Design review of the part built by this model. Coordinates are the model's own, in mm. A direction names the side the tool comes from. Give positions to 0.01 mm unless a question says otherwise; leave off trailing zeros. Loops run counter-clockwise (first coordinate to the right, second up) from the corner with the lowest first, then second, coordinate; pieces in that order, holes last. Notation, with made-up numbers: (45.25, 36) - (78.25, 36) arc R21 cw to (78.25, 57) - close; hole circle Ø4 at (24.5, 75). An arc over 180 degrees is marked (long way). Write each question's results on one line, items separated by ' | '.
```python
from build123d import *

# Parameters (mm, degrees)
BOSS_EXTRUDE1_DEPTH      = 20
BOSS_EXTRUDE2_DEPTH      = 65
BOSS_EXTRUDE2_DEPTH_BACK = 20
SKETCH3_R                = 31
SKETCH3_R_2              = 12.5
SKETCH6_R                = 20
CUT_EXTRUDE1_DEPTH       = 26
SKETCH8_R                = 12.5
CUT_EXTRUDE2_DEPTH       = 20
SKETCH9_R                = 3
CUT_EXTRUDE3_DEPTH       = 33


with BuildPart() as part:
    # Sketch2 → Boss-Extrude1 (new body)
    with BuildSketch(Plane.XY):
        with BuildLine():
            Line((0, 0), (56.291651246, -32.5))
            ThreePointArc((56.291651246, -32.5), (64.9518339, -2.501853916), (58.624860802, 28.073576473))
            Line((58.624860802, 28.073576473), (45.634479745, 20.573576473))
            Line((45.634479745, 20.573576473), (40.634479745, 29.233830511))
            Line((40.634479745, 29.233830511), (53.624860802, 36.733830511))
            ThreePointArc((53.624860802, 36.733830511), (32.5, 56.291651246), (5, 64.807406984))
            Line((5, 64.807406984), (5, 49.807406984))
            Line((5, 49.807406984), (-5, 49.807406984))
            Line((-5, 49.807406984), (-5, 64.807406984))
            ThreePointArc((-5, 64.807406984), (-32.5, 56.291651246), (-53.624860802, 36.733830511))
            Line((-53.624860802, 36.733830511), (-40.634479745, 29.233830511))
            Line((-40.634479745, 29.233830511), (-45.634479745, 20.573576473))
            Line((-45.634479745, 20.573576473), (-58.624860802, 28.073576473))
            ThreePointArc((-58.624860802, 28.073576473), (-64.9518339, -2.501853916), (-56.291651246, -32.5))
            Line((-56.291651246, -32.5), (0, 0))
        make_face()
    extrude(amount=BOSS_EXTRUDE1_DEPTH)

    # Sketch3 → Boss-Extrude2 (add, two sides: drawn at the far end of the back side and taken through both)
    with BuildSketch(Plane.XY.offset(20).offset(-BOSS_EXTRUDE2_DEPTH_BACK)):
        Circle(SKETCH3_R)
        Circle(SKETCH3_R_2, mode=Mode.SUBTRACT)
    extrude(amount=BOSS_EXTRUDE2_DEPTH + BOSS_EXTRUDE2_DEPTH_BACK)

    # Cut-Sweep1: sweep along a curve in space
    with BuildLine() as cut_sweep1_path:
        ThreePointArc((31, 0, 85), (21.920310217, 21.920310217, 85), (0, 31, 85))
        ThreePointArc((0, 31, 85), (-21.920310217, 21.920310217, 85), (-31, 0, 85))
        ThreePointArc((-31, 0, 85), (-21.920310217, -21.920310217, 85), (0, -31, 85))
        ThreePointArc((0, -31, 85), (21.920310217, -21.920310217, 85), (31, 0, 85))
    # Sketch5 → Cut-Sweep1 (sweep, cut)
    with BuildSketch(Plane(origin=(0, 0, 0), x_dir=(0, 0, -1), z_dir=(1, 0, 0))):
        Polygon((-85, 31), (-73, 31), (-85, 24.07179677), align=None)
    sweep(path=cut_sweep1_path.line, mode=Mode.SUBTRACT)

    # Sketch6 → Cut-Extrude1 (cut)
    with BuildSketch(Plane.XY.offset(85)):
        Circle(SKETCH6_R)
    extrude(amount=-CUT_EXTRUDE1_DEPTH, mode=Mode.SUBTRACT)

    # Sketch8 → Cut-Extrude2 (cut)
    with BuildSketch(Plane.XY.offset(20)):
        Circle(SKETCH8_R)
    extrude(amount=-CUT_EXTRUDE2_DEPTH, mode=Mode.SUBTRACT)

    # Sketch9 → Cut-Extrude3 (cut)
    with BuildSketch(Plane(origin=(0, 0, 0), x_dir=(1, 0, 0), z_dir=(0, 1, 0))):
        with Locations(Location((0, -33, 0), (0, 0, 90))):
            Circle(SKETCH9_R)
    extrude(amount=CUT_EXTRUDE3_DEPTH, mode=Mode.SUBTRACT)


solid = part.part
```
Item 1: Draft analysis for pull direction X (two halves, no side actions). For faces 1 (the face through (-15, 28, 20)), 2 (the face through (-32.15, 56.49, 9.86)), 3 (the face through (-43.1, 24.96, 9.86)), state which applies: +X half, -X half, draft (parallel to the pull), parting line (faces both ways), or undercut.
Output values:
face 1: draft | face 2: -X half | face 3: undercut
Item 2: Wall thickness on probe 1 along X at (y, z) = (-18.5, 17); probe 2 along Y at (x, z) = (0, 14); probe 3 along Z at (x, y) = (45, 1): over which ranges is each line inside the solid? List them lowest first.
Output values:
probe 1: x = -62.31 to -32.04, -24.87 to 24.87, 32.04 to 62.31 | probe 2: y = -31 to -12.5, 12.5 to 49.81 | probe 3: z = 0 to 20
Item 3: Tool access review of faces 4 (the face through (-4.336, -19.524, 72.182)), 5 (the face through (41.4, -23.9, 9.9)), 6 (the face through (52.221, 24.376, 9.86)): name each direction out of +Z, -Z, +X, -X, +Y, -Y from which nothing blocks a thin tool from reaching the whole face with its end or side.
Output values:
face 4: +Z | face 5: +Z, -Z, -Y | face 6: +Z, -Z
Item 4: We need section A-A on z = 7. Give the boundary of the cut face in (x, y).
Output values:
outline: (-58.62, 28.07) arc R65 ccw to (-56.29, -32.5) - (-26.85, -15.5) arc R31 ccw to (26.85, -15.5) - (56.29, -32.5) arc R65 ccw to (58.62, 28.07) - (45.63, 20.57) - (40.63, 29.23) - (53.62, 36.73) arc R65 ccw to (5, 64.81) - (5, 49.81) - (-5, 49.81) - (-5, 64.81) arc R65 ccw to (-53.62, 36.73) - (-40.63, 29.23) - (-45.63, 20.57) - close; hole circle Ø25 at (0, 0)
Item 5: Clearance check with flat-ended pins moving along their axes: P1, Ø8, axis at x = -35.5, y = 10.5, coming from the +Z side; P2, Ø8, axis at x = -2.5, z = 12.5, coming from the +Y side; P3, Ø16.5, axis at y = 59, z = 12, coming from the -X side. State where each tip first meets the part, or that it passes through.
Output values:
P1: stops at z = 20 | P2: stops at y = 64.81 | P3: stops at x = -40.61
Item 6: We need section B-B on x = -51. Give the boundary of the cut face in (y, z), then the cut area to 3 significant figures.
Output values:
outline: (-29.44, 0) - (23.67, 0) - (23.67, 20) - (-29.44, 20) - close; (35.22, 0) - (40.3, 0) - (40.3, 20) - (35.22, 20) - close | area: 1,160 mm²
Item 7: We need section D-D on x = 38. Give the boundary of the cut face in (y, z), then the cut area to 3 significant figures.
Output values:
outline: (-21.94, 0) - (52.74, 0) - (52.74, 20) - (-21.94, 20) - close | area: 1,490 mm²
Item 8: We need section C-C on y = 53. Give the boundary of the cut face in (x, z), then the cut area to 3 significant figures.
Output values:
outline: (-37.63, 0) - (-5, 0) - (-5, 20) - (-37.63, 20) - close; (5, 0) - (37.63, 0) - (37.63, 20) - (5, 20) - close | area: 1,310 mm²
